Geometry check sheet. Reference: the model listing, model coordinates, mm. Face numbers are marked on the shaded views. A direction names the side the tool comes from. Round coordinates to 2 decimals unless told otherwise and drop trailing zeros. Order: outer loops, then holes, each group sorted by start corner. A loop starts at its lowest first (then second) coordinate and runs counter-clockwise, first axis right, second up.
(1) Draft check along X on the marked faces 1, 2 and 3. Enter one of: pulls with the +X half, pulls with the -X half, needs draft (parallel to the pull), parting line crosses it, or undercut.
(2) Gauge pin test, flat ends, axial feed: P1, Ø1.8, axis at x = 25, y = 3, coming from the +Z side; P2, Ø3, axis at x = 18, y = 4, coming from the +Z side; P3, Ø3, axis at x = -22.5, y = 3.5, coming from the -Z side. Record the tip position at first contact, or that the pin passes through.
(3) Cross-section at D-D on z = -4.75. Enter the section's corners in (x, y).
(4) Cross-section at C-C on x = -12. Enter the section's corners in (y, z).
(5) Set-up check for the marked faces 4, 5 and 6: record each of +Z, -Z, +X, -X, +Y, -Y from which the full face is reachable in a straight line by a thin tool's end or side.
(6) Thickness scan on L1, parallel to X at y = 4.5, z = 5.5; L2, parallel to X at y = 4.5, z = 8.5; L3, parallel to X at y = 3, z = -2. Record the ranges inside material, lowest first.
(7) Cross-section at A-A on z = 4.75. Enter the section's corners in (x, y).
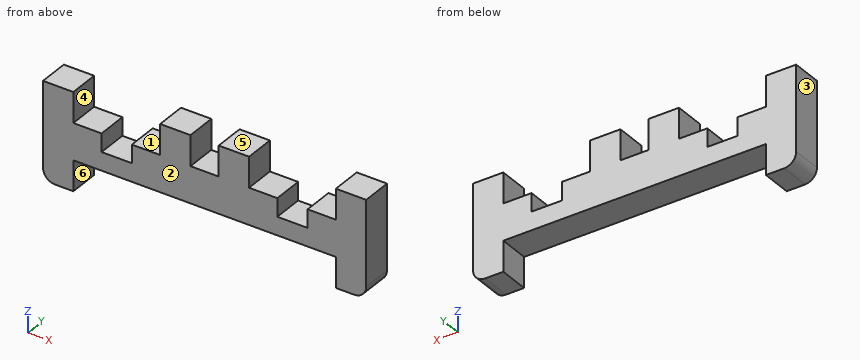
from build123d import *

# Parameters (mm, degrees)
BOSS_EXTRUDE1_DEPTH = 6.35


with BuildPart() as part:
    # Sketch1 → Boss-Extrude1 (new body)
    with BuildSketch(Plane(origin=(0, 0, 0), x_dir=(1, 0, 0), z_dir=(0, 1, 0))):
        with BuildLine():
            Line((-24.3205, 0), (24.3205, 0))
            Line((24.3205, 0), (27.4955, 0))
            Line((27.4955, 0), (27.4955, 6.35))
            Line((27.4955, 6.35), (31.3055, 6.35))
            ThreePointArc((31.3055, 6.35), (33.101551224, 5.606051224), (33.8455, 3.81))
            Line((33.8455, 3.81), (33.8455, -13.97))
            Line((33.8455, -13.97), (27.4955, -13.97))
            Line((27.4955, -13.97), (27.4955, -7.62))
            Line((27.4955, -7.62), (21.5773, -7.62))
            Line((21.5773, -7.62), (21.5773, -3.81))
            Line((21.5773, -3.81), (15.2273, -3.81))
            Line((15.2273, -3.81), (15.2273, -7.62))
            Line((15.2273, -7.62), (9.3091, -7.62))
            Line((9.3091, -7.62), (9.3091, -13.97))
            Line((9.3091, -13.97), (2.9591, -13.97))
            Line((2.9591, -13.97), (2.9591, -7.62))
            Line((2.9591, -7.62), (-2.9591, -7.62))
            Line((-2.9591, -7.62), (-2.9591, -13.97))
            Line((-2.9591, -13.97), (-9.3091, -13.97))
            Line((-9.3091, -13.97), (-9.3091, -7.62))
            Line((-9.3091, -7.62), (-15.2273, -7.62))
            Line((-15.2273, -7.62), (-15.2273, -3.81))
            Line((-15.2273, -3.81), (-21.5773, -3.81))
            Line((-21.5773, -3.81), (-21.5773, -7.62))
            Line((-21.5773, -7.62), (-27.4955, -7.62))
            Line((-27.4955, -7.62), (-27.4955, -13.97))
            Line((-27.4955, -13.97), (-33.8455, -13.97))
            Line((-33.8455, -13.97), (-33.8455, -7.62))
            Line((-33.8455, -7.62), (-33.8455, 3.81))
            ThreePointArc((-33.8455, 3.81), (-33.101551224, 5.606051224), (-31.3055, 6.35))
            Line((-31.3055, 6.35), (-27.4955, 6.35))
            Line((-27.4955, 6.35), (-27.4955, 0))
            Line((-27.4955, 0), (-24.3205, 0))
        make_face()
    extrude(amount=BOSS_EXTRUDE1_DEPTH)


solid = part.part
Found:
1. face 1: undercut
1. face 2: needs draft
1. face 3: pulls with the -X half
2. P1: stops at z = 7.62
2. P2: stops at z = 3.81
2. P3: stops at z = 0
3. outline: (-33.67, 0) - (-27.5, 0) - (-27.5, 6.35) - (-33.67, 6.35) - close; (27.5, 0) - (33.67, 0) - (33.67, 6.35) - (27.5, 6.35) - close
4. outline: (0, 0) - (6.35, 0) - (6.35, 7.62) - (0, 7.62) - close
5. face 4: +Z, +Y, -Y
5. face 5: +Z, +X, -X, +Y, -Y
5. face 6: -Z, +Y, -Y
6. L1: x = -33.85 to -21.58, -15.23 to 15.23, 21.58 to 33.85
6. L2: x = -33.85 to -27.5, -9.31 to -2.96, 2.96 to 9.31, 27.5 to 33.85
6. L3: x = -33.85 to -27.5, 27.5 to 33.85
7. outline: (-33.85, 0) - (-21.58, 0) - (-21.58, 6.35) - (-33.85, 6.35) - close; (-15.23, 0) - (15.23, 0) - (15.23, 6.35) - (-15.23, 6.35) - close; (21.58, 0) - (33.85, 0) - (33.85, 6.35) - (21.58, 6.35) - close
